Can you work these out from the model? Positions are in its coordinate system, mm. Face numbers are marked on the shaded views. Give positions to 0.01 mm unless a question says otherwise; leave off trailing zeros. Loops run counter-clockwise (first coordinate to the right, second up) from the corner with the lowest first, then second, coordinate; pieces in that order, holes last. Notation, with made-up numbers: (39.25, -25.5) - (79.25, -25.5) arc R19 ccw to (79.25, -21.5) - close; hole circle Ø3 at (64.5, 1). An arc over 180 degrees is marked (long way). Answer as a JSON object with one key per item and string values.
```python
from build123d import *

# Parameters (mm, degrees)
SKETCH1_W                                            = 96
SKETCH1_H                                            = 120
BOSS_EXTRUDE1_DEPTH                                  = 8
CSK_FOR_M6_HEX_SOCKET_COUNTERSUNK_CAP_SC_D           = 6.6
CSK_FOR_M6_HEX_SOCKET_COUNTERSUNK_CAP_SC_CSINK_D     = 13.44
CSK_FOR_M6_HEX_SOCKET_COUNTERSUNK_CAP_SC_CSINK_ANGLE = 90
SKETCH4_W                                            = 15
SKETCH4_H                                            = 120
BOSS_EXTRUDE2_DEPTH                                  = 25
M6_TAPPED_HOLE1_D                                    = 5
SKETCH8_W                                            = 96
SKETCH8_H                                            = 47
BOSS_EXTRUDE4_DEPTH                                  = 8
M5_TAPPED_HOLE1_D                                    = 4.2
CSK_FOR_M6_HEX_SOCKET_COUNTERSUNK_CA_2_A_COUNT       = 2
CSK_FOR_M6_HEX_SOCKET_COUNTERSUNK_CA_2_A_PITCH       = 60
SKETCH16_W                                           = 2.5
SKETCH16_H                                           = 25
M6_TAPPED_HOLE2_AT_2_COUNT                           = 2
M6_TAPPED_HOLE2_AT_2_PITCH                           = 60


# Read off the part's stored shape, not the designer's step: Split1
with BuildPart() as part:
    # Sketch1 → Boss-Extrude1 (new body)
    with BuildSketch(Plane.XY):
        Rectangle(SKETCH1_W, SKETCH1_H)
    extrude(amount=BOSS_EXTRUDE1_DEPTH)

    # CSK for M6 Hex Socket Countersunk Cap Sc (through all)
    with Locations(Plane.XY.offset(8)):
        with Locations((-35, 53), (-35, 13), (-35, -8), (-35, -48)):
            csk_for_m6_hex_socket_countersunk_cap_sc = CounterSinkHole(CSK_FOR_M6_HEX_SOCKET_COUNTERSUNK_CAP_SC_D / 2, CSK_FOR_M6_HEX_SOCKET_COUNTERSUNK_CAP_SC_CSINK_D / 2, counter_sink_angle=CSK_FOR_M6_HEX_SOCKET_COUNTERSUNK_CAP_SC_CSINK_ANGLE)

    # Sketch4 → Boss-Extrude2 (add)
    with BuildSketch(Plane.XY.offset(8)):
        with Locations((12.5, 0)):
            Rectangle(SKETCH4_W, SKETCH4_H)
    extrude(amount=BOSS_EXTRUDE2_DEPTH)

    # M6 Tapped Hole1 (through all)
    with Locations(Plane.ZY.offset(-5)):
        with Locations((20.5, -40), (20.5, 40)):
            Hole(M6_TAPPED_HOLE1_D / 2)

    # Sketch8 → Boss-Extrude4 (add)
    with BuildSketch(Plane.XY.offset(8)):
        with Locations((0, 83.5)):
            Rectangle(SKETCH8_W, SKETCH8_H)
    extrude(amount=-BOSS_EXTRUDE4_DEPTH)

    # M5 Tapped Hole1 (through all)
    with Locations(Plane.XY.offset(8)):
        with Locations((-43, 101), (-43, 75), (-18, 101), (-18, 75), (18, 75), (18, 101), (43, 101), (43, 75)):
            Hole(M5_TAPPED_HOLE1_D / 2)

    # Mirror1: CSK for M6 Hex Socket Countersunk Cap Sc across plane
    add(csk_for_m6_hex_socket_countersunk_cap_sc.mirror(Plane(origin=(0, 0, 0), x_dir=(0, 0, 1), z_dir=(1, 0, 0))), mode=Mode.SUBTRACT)


with BuildPart() as body_2:
    # Split1: the piece on the far side of the plane
    add(part.part)
    split(bisect_by=Plane.XY.offset(8), keep=Keep.BOTTOM)

    # Sketch14 → CSK for M6 Hex Socket Countersunk Ca 2 (revolve, cut)
    with BuildSketch(Plane(origin=(12.5, 30, 0), x_dir=(0, 1, 0), z_dir=(1, 0, 0))):
        Polygon((0, 0), (0, 33), (3.3, 33), (3.3, 3.92), (7.22, 0), align=None)
    csk_for_m6_hex_socket_countersunk_ca_2 = revolve(axis=Axis((12.5, 30, -6.35), (0, 0, 1)), mode=Mode.SUBTRACT)

    # CSK for M6 Hex Socket Countersunk Ca 2 a: CSK for M6 Hex Socket Countersunk Ca 2 ×2
    with Locations(*[(0, -i * CSK_FOR_M6_HEX_SOCKET_COUNTERSUNK_CA_2_A_PITCH, 0) for i in range(1, CSK_FOR_M6_HEX_SOCKET_COUNTERSUNK_CA_2_A_COUNT)]):
        add(csk_for_m6_hex_socket_countersunk_ca_2, mode=Mode.SUBTRACT)


with BuildPart() as part_1:
    add(part.part)

    # Split1
    split(bisect_by=Plane.XY.offset(8), keep=Keep.TOP)

    # Sketch16 → M6 Tapped Hole2 (revolve, cut)
    with BuildSketch(Plane(origin=(12.5, 30, 8), x_dir=(0, 1, 0), z_dir=(1, 0, 0))):
        with Locations((1.25, 12.5)):
            Rectangle(SKETCH16_W, SKETCH16_H)
    m6_tapped_hole2 = revolve(axis=Axis((12.5, 30, 1.65), (0, 0, 1)), mode=Mode.SUBTRACT)

    # M6 Tapped Hole2 at 2: M6 Tapped Hole2 ×2
    with Locations(*[(0, -i * M6_TAPPED_HOLE2_AT_2_PITCH, 0) for i in range(1, M6_TAPPED_HOLE2_AT_2_COUNT)]):
        add(m6_tapped_hole2, mode=Mode.SUBTRACT)


solid = body_2.part
```
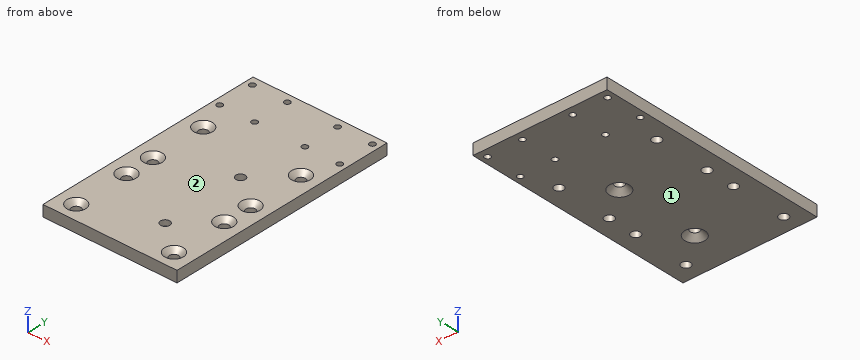
1) Imagine slicing it at C-C on z = 2. Give the number of separate pieces and of enclosed holes in the cut face, and give its area (3 significant figures).
Check sheet entries:
{"separate pieces": "1", "enclosed holes": "18", "area": "15,500 mm2"}
2) Imagine slicing it at A-A on x = -18. Write out the boundary of the cut face in (y, z).
Check sheet entries:
{"outline": "(-60, 0) - (72.9, 0) - (72.9, 8) - (-60, 8) - close; (77.1, 0) - (98.9, 0) - (98.9, 8) - (77.1, 8) - close; (103.1, 0) - (107, 0) - (107, 8) - (103.1, 8) - close"}
3) If we mould it in two halves opening along Z, with no side actions, what happens to the marked faces 1 and 2? For each: released by +Z, released by -Z, zero draft, split by the parting line, or undercut.
Check sheet entries:
{"face 1": "released by -Z", "face 2": "released by +Z"}
4) I need wall thicknesses on L1, parallel to X at y = 13, z = 1; L2, parallel to Y at x = -35, z = 3.6; L3, parallel to Y at x = 12.5, z = 5.5. Which ranges of each line are inside material? Lowest first, please.
Check sheet entries:
{"L1": "-48 to -38.3, -31.7 to 31.7, 38.3 to 48", "L2": "-60 to -51.3, -44.7 to -11.3, -4.7 to 9.7, 16.3 to 49.7, 56.3 to 107", "L3": "-60 to -33.3, -26.7 to 26.7, 33.3 to 107"}
5) Imagine slicing it at B-B on y = 53. Write out the boundary of the cut face in (x, z).
Check sheet entries:
{"outline": "(-48, 0) - (-38.3, 0) - (-38.3, 4.58) - (-41.72, 8) - (-48, 8) - close; (-31.7, 0) - (31.7, 0) - (31.7, 4.58) - (28.28, 8) - (-28.28, 8) - (-31.7, 4.58) - close; (38.3, 0) - (48, 0) - (48, 8) - (41.72, 8) - (38.3, 4.58) - close"}
